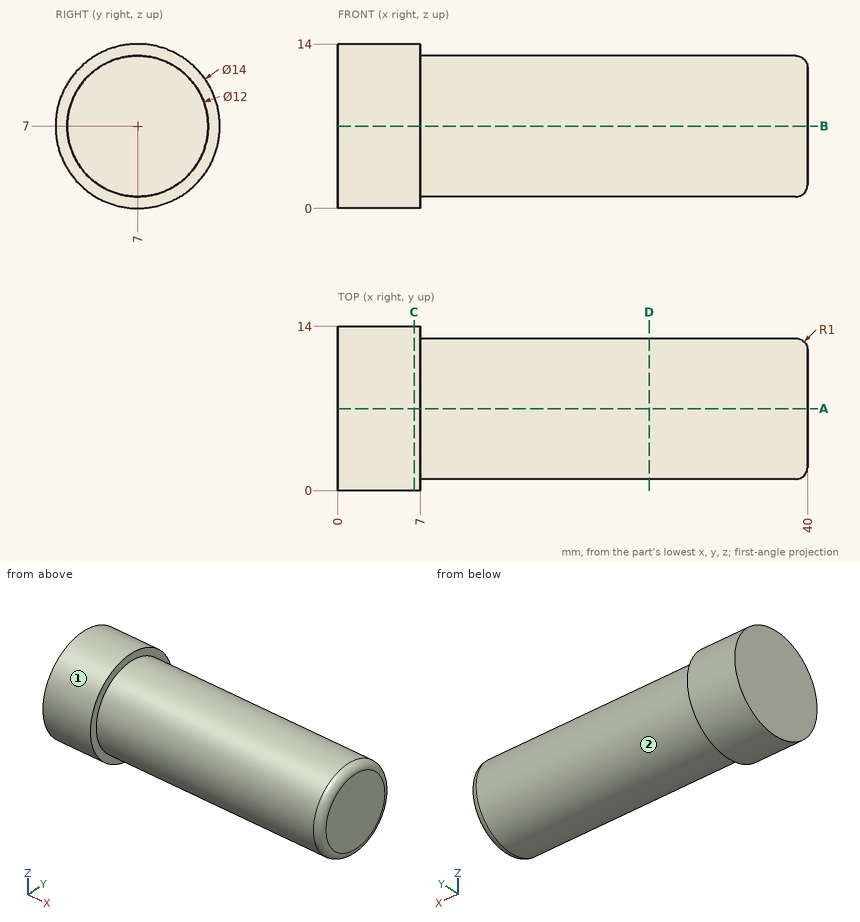
Design review of the part shown in the three views and the two pictorial views. Dimensions are in mm from the part's minimum x, y and z. A direction names the side the tool comes from. Round coordinates to 2 decimals unless told otherwise and drop trailing zeros. Order: outer loops, then holes, each group sorted by start corner. A loop starts at its lowest first (then second) coordinate and runs counter-clockwise, first axis right, second up.
(1) Wall thickness on L1, parallel to X at y = 1.5, z = 10; L2, parallel to X at y = 2.25, z = 4.5; L3, parallel to Z at x = 37.5, y = 5.75: over which ranges is each line inside the solid? List them lowest first.
Working result:
L1: x = 0 to 7
L2: x = 0 to 39.93
L3: z = 1.13 to 12.87
(2) Take a section at A-A, the plane y = 7. State the section outline as (x, z) points.
Working result:
outline: (0, 0) - (7, 0) - (7, 1) - (39, 1) arc R1 ccw to (40, 2) - (40, 12) arc R1 ccw to (39, 13) - (7, 13) - (7, 14) - (0, 14) - close
(3) For P1, Ø1.5, axis at x = 21, y = 10.5, coming from the -Z side; P2, Ø2, axis at x = 24.5, y = 5, coming from the -Z side; P3, Ø2, axis at x = 35, z = 6, coming from the -Y side, all flat-tipped, find the tip position at first contact; note any pin that passes through.
Working result:
P1: stops at z = 1.67
P2: stops at z = 1.08
P3: stops at y = 1
(4) Tool access review of the marked faces 1 and 2: name each direction out of +Z, -Z, +X, -X, +Y, -Y from which nothing blocks a thin tool from reaching the whole face with its end or side.
Working result:
face 1: +X, -X
face 2: +X
(5) Take a section at C-C, the plane x = 6.5. State the section outline as (y, z) points, plus the area to 3 significant figures.
Working result:
outline: circle Ø14 at (7, 7)
area: 154 mm2
(6) Take a section at D-D, the plane x = 26.5. State the section outline as (y, z) points.
Working result:
outline: circle Ø12 at (7, 7)
